Can you work these out from the model? Positions are in its coordinate system, mm. Face numbers are marked on the shaded views. Coordinates: 2 decimals unless noted, no trailing zeros. Write each loop counter-clockwise with the first axis right and the second up, starting at its lowest first coordinate (ties: lowest second). Pieces come first, ordered by that corner, then holes. Notation, with made-up numbers: (-31.5, -13) -> (-2.5, -13) arc R7 ccw to (-2.5, -8) -> close; hole circle Ø3 at (5, 62). An arc over 180 degrees is marked (long way). Use one line per item in the form item = value.
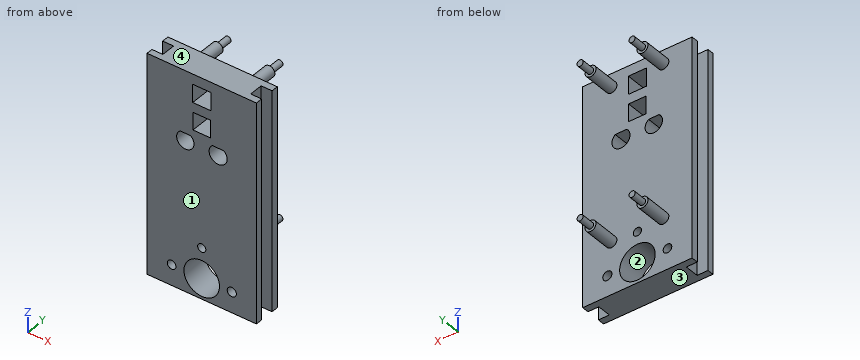
```python
from build123d import *

# Parameters (mm, degrees)
ESQUISSE2_W             = 40
ESQUISSE2_H             = 80
BOSS_EXTRU_1_DEPTH      = 10
ESQUISSE3_R             = 2
BOSS_EXTRU_2_DEPTH      = 10
ESQUISSE4_R             = 1.125
BOSS_EXTRU_3_DEPTH      = 5
ENL_V_MAT_EXTRU_1_REACH = 49.17
ESQUISSE5_R             = 1.5
ESQUISSE5_R_2           = 1.575
ESQUISSE5_R_3           = 1.675
ESQUISSE5_R_4           = 6.5
ENL_V_MAT_EXTRU_2_REACH = 49.17
ESQUISSE6_W             = 6.6
ESQUISSE6_H             = 6.6
ESQUISSE6_W_2           = 6.4
ESQUISSE6_H_2           = 6.4
ENL_V_MAT_EXTRU_3_DEPTH = 10
ENL_V_MAT_EXTRU_4_REACH = 88.168
ESQUISSE8_W             = 4
ESQUISSE8_H             = 5
ESQUISSE8_H_2           = 5.15


with BuildPart() as part:
    # Esquisse2 → Boss.-Extru.1 (new body)
    with BuildSketch(Plane(origin=(0, 0, 0), x_dir=(1, 0, 0), z_dir=(0, 1, 0))):
        Rectangle(ESQUISSE2_W, ESQUISSE2_H)
    extrude(amount=BOSS_EXTRU_1_DEPTH)

    # Esquisse3 → Boss.-Extru.2 (add)
    with BuildSketch(Plane(origin=(0, 10, 0), x_dir=(1, 0, 0), z_dir=(0, 1, 0))):
        with Locations(Location((9.5, -35, 0), (0, 0, 270))):
            Circle(ESQUISSE3_R)
        with Locations(Location((9.5, 21, 0), (0, 0, 270))):
            Circle(ESQUISSE3_R)
        with Locations(Location((-9.5, -35, 0), (0, 0, 270))):
            Circle(ESQUISSE3_R)
        with Locations(Location((-9.5, 21, 0), (0, 0, 270))):
            Circle(ESQUISSE3_R)
    extrude(amount=BOSS_EXTRU_2_DEPTH)

    # Esquisse4 → Boss.-Extru.3 (add)
    with BuildSketch(Plane(origin=(0, 20, 0), x_dir=(1, 0, 0), z_dir=(0, 1, 0))):
        with Locations(Location((-9.5, -35, 0), (0, 0, 270))):
            Circle(ESQUISSE4_R)
        with Locations(Location((9.5, -35, 0), (0, 0, 270))):
            Circle(ESQUISSE4_R)
        with Locations(Location((-9.5, 21, 0), (0, 0, 270))):
            Circle(ESQUISSE4_R)
        with Locations(Location((9.5, 21, 0), (0, 0, 270))):
            Circle(ESQUISSE4_R)
    extrude(amount=BOSS_EXTRU_3_DEPTH)

    # Esquisse5 → Enlèv. mat.-Extru.1 (cut, up to next)
    with BuildSketch(Plane(origin=(0, 10, 0), x_dir=(1, 0, 0), z_dir=(0, 1, 0)), mode=Mode.PRIVATE) as enl_v_mat_extru_1_sk1:
        with Locations(Location((0, 21.5, 0), (0, 0, 270))):
            Circle(ESQUISSE5_R)
    enl_v_mat_extru_1_tool1 = extrude(enl_v_mat_extru_1_sk1.sketch, amount=-ENL_V_MAT_EXTRU_1_REACH, mode=Mode.PRIVATE) & part.part
    # Esquisse5 → Enlèv. mat.-Extru.1 (cut, up to next)
    with BuildSketch(Plane(origin=(0, 10, 0), x_dir=(1, 0, 0), z_dir=(0, 1, 0)), mode=Mode.PRIVATE) as enl_v_mat_extru_1_sk2:
        with Locations(Location((-11, 32.5, 0), (0, 0, 270))):
            Circle(ESQUISSE5_R_2)
    enl_v_mat_extru_1_tool2 = extrude(enl_v_mat_extru_1_sk2.sketch, amount=-ENL_V_MAT_EXTRU_1_REACH, mode=Mode.PRIVATE) & part.part
    # Esquisse5 → Enlèv. mat.-Extru.1 (cut, up to next)
    with BuildSketch(Plane(origin=(0, 10, 0), x_dir=(1, 0, 0), z_dir=(0, 1, 0)), mode=Mode.PRIVATE) as enl_v_mat_extru_1_sk3:
        with Locations(Location((11, 32.5, 0), (0, 0, 270))):
            Circle(ESQUISSE5_R_3)
    enl_v_mat_extru_1_tool3 = extrude(enl_v_mat_extru_1_sk3.sketch, amount=-ENL_V_MAT_EXTRU_1_REACH, mode=Mode.PRIVATE) & part.part
    # Esquisse5 → Enlèv. mat.-Extru.1 (cut, up to next)
    with BuildSketch(Plane(origin=(0, 10, 0), x_dir=(1, 0, 0), z_dir=(0, 1, 0)), mode=Mode.PRIVATE) as enl_v_mat_extru_1_sk4:
        with Locations(Location((0, 32.5, 0), (0, 0, 270))):
            Circle(ESQUISSE5_R_4)
    enl_v_mat_extru_1_tool4 = extrude(enl_v_mat_extru_1_sk4.sketch, amount=-ENL_V_MAT_EXTRU_1_REACH, mode=Mode.PRIVATE) & part.part
    add(enl_v_mat_extru_1_tool1.solids().sort_by_distance((0, 10, -21.5))[0], mode=Mode.SUBTRACT)
    add(enl_v_mat_extru_1_tool2.solids().sort_by_distance((-11, 10, -32.5))[0], mode=Mode.SUBTRACT)
    add(enl_v_mat_extru_1_tool3.solids().sort_by_distance((11, 10, -32.5))[0], mode=Mode.SUBTRACT)
    add(enl_v_mat_extru_1_tool4.solids().sort_by_distance((0, 10, -32.5))[0], mode=Mode.SUBTRACT)

    # Esquisse6 → Enlèv. mat.-Extru.2 (cut, up to next)
    with BuildSketch(Plane(origin=(0, 10, 0), x_dir=(1, 0, 0), z_dir=(0, 1, 0)), mode=Mode.PRIVATE) as enl_v_mat_extru_2_sk1:
        with Locations((0, -33)):
            Rectangle(ESQUISSE6_W, ESQUISSE6_H)
    enl_v_mat_extru_2_tool1 = extrude(enl_v_mat_extru_2_sk1.sketch, amount=-ENL_V_MAT_EXTRU_2_REACH, mode=Mode.PRIVATE) & part.part
    # Esquisse6 → Enlèv. mat.-Extru.2 (cut, up to next)
    with BuildSketch(Plane(origin=(0, 10, 0), x_dir=(1, 0, 0), z_dir=(0, 1, 0)), mode=Mode.PRIVATE) as enl_v_mat_extru_2_sk2:
        with Locations((0, -23)):
            Rectangle(ESQUISSE6_W_2, ESQUISSE6_H_2)
    enl_v_mat_extru_2_tool2 = extrude(enl_v_mat_extru_2_sk2.sketch, amount=-ENL_V_MAT_EXTRU_2_REACH, mode=Mode.PRIVATE) & part.part
    add(enl_v_mat_extru_2_tool1.solids().sort_by_distance((0, 10, 33))[0], mode=Mode.SUBTRACT)
    add(enl_v_mat_extru_2_tool2.solids().sort_by_distance((0, 10, 23))[0], mode=Mode.SUBTRACT)

    # Esquisse7 → Enlèv. mat.-Extru.3 (cut)
    with BuildSketch(Plane(origin=(0, 10, 0), x_dir=(1, 0, 0), z_dir=(0, 1, 0))):
        with BuildLine():
            Line((-7.905, -17.34), (-4.095, -17.34))
            ThreePointArc((-4.095, -17.34), (-6, -11.625), (-7.905, -17.34))
        make_face()
        with BuildLine():
            Line((3.890117539, -17.34), (8.109882461, -17.34))
            ThreePointArc((8.109882461, -17.34), (6, -11.498), (3.890117539, -17.34))
        make_face()
    extrude(amount=-ENL_V_MAT_EXTRU_3_DEPTH, mode=Mode.SUBTRACT)

    # Esquisse8 → Enlèv. mat.-Extru.4 (cut, up to next)
    with BuildSketch(Plane.XY.offset(40), mode=Mode.PRIVATE) as enl_v_mat_extru_4_sk1:
        with Locations((18, 5)):
            Rectangle(ESQUISSE8_W, ESQUISSE8_H)
    enl_v_mat_extru_4_tool1 = extrude(enl_v_mat_extru_4_sk1.sketch, amount=-ENL_V_MAT_EXTRU_4_REACH, mode=Mode.PRIVATE) & part.part
    # Esquisse8 → Enlèv. mat.-Extru.4 (cut, up to next)
    with BuildSketch(Plane.XY.offset(40), mode=Mode.PRIVATE) as enl_v_mat_extru_4_sk2:
        with Locations((-18, 4.925)):
            Rectangle(ESQUISSE8_W, ESQUISSE8_H_2)
    enl_v_mat_extru_4_tool2 = extrude(enl_v_mat_extru_4_sk2.sketch, amount=-ENL_V_MAT_EXTRU_4_REACH, mode=Mode.PRIVATE) & part.part
    add(enl_v_mat_extru_4_tool1.solids().sort_by_distance((18, 5, 40))[0], mode=Mode.SUBTRACT)
    add(enl_v_mat_extru_4_tool2.solids().sort_by_distance((-18, 4.925, 40))[0], mode=Mode.SUBTRACT)


solid = part.part
```
Q1. Thinking about a two-plate mould opening in Z: for the marked faces 1, 2, 3 and 4, which applies, released by +Z, released by -Z, zero draft, split by the parting line, or undercut?
Return value:
face_1 = zero draft
face_2 = undercut
face_3 = released by -Z
face_4 = released by +Z
Q2. Will these pins go through, and if not, where does the flat tip stop? pin 1 (1.5 mm diameter, centred on x = -12, z = 15.5, fed in from -Y); pin 2 (3.5 mm diameter, centred on x = -11, z = -32.5, fed in from +Y); pin 3 (3.5 mm diameter, centred on y = 5, z = 32, fed in from +X); pin 4 (4 mm diameter, centred on x = 11.5, y = 18, fed in from +Z).
Return value:
pin_1 = 0
pin_2 = 10
pin_3 = 16
pin_4 = 37
Q3. Suppose I cut it at D-D (z = -32.5). Write out the boundary of the cut face in (x, y) (3 decimals), then the cut area to 3 significant figures.
Return value:
outline = (-20, 0) -> (-12.575, 0) -> (-12.575, 10) -> (-20, 10) -> (-20, 7.5) -> (-16, 7.5) -> (-16, 2.35) -> (-20, 2.35) -> close; (-9.425, 0) -> (-6.5, 0) -> (-6.5, 10) -> (-9.425, 10) -> close; (6.5, 0) -> (9.325, 0) -> (9.325, 10) -> (6.5, 10) -> close; (12.675, 0) -> (20, 0) -> (20, 2.5) -> (16, 2.5) -> (16, 7.5) -> (20, 7.5) -> (20, 10) -> (12.675, 10) -> close
area = 164 mm2
Q4. If I drill on line 1 (X direction, y = 6.25, z = 14.8) (3 decimals); line 2 (X direction, y = 4.25, z = -21.5); line 3 (Z direction, x = 6, y = 8), over which ranges is the centre line in solid material (lowest first)? Write a range as from..to.
Return value:
line_1 = -16..-9.175, -2.825..2.698, 9.302..16
line_2 = -16..-1.5, 1.5..16
line_3 = -40..-35, -30..11.5, 17.34..40
Q5. Suppose I cut it at A-A (x = 0). Write out the boundary of the cut face in (y, z).
Return value:
outline = (0, -40) -> (10, -40) -> (10, -39) -> (0, -39) -> close; (0, -26) -> (10, -26) -> (10, -23) -> (0, -23) -> close; (0, -20) -> (10, -20) -> (10, 19.8) -> (0, 19.8) -> close; (0, 26.2) -> (10, 26.2) -> (10, 29.7) -> (0, 29.7) -> close; (0, 36.3) -> (10, 36.3) -> (10, 40) -> (0, 40) -> close
Q6. Suppose I cut it at B-B (x = 17). Write out the boundary of the cut face in (y, z), then the cut area to 3 significant figures.
Return value:
outline = (0, -40) -> (2.5, -40) -> (2.5, 40) -> (0, 40) -> close; (7.5, -40) -> (10, -40) -> (10, 40) -> (7.5, 40) -> close
area = 400 mm2
